Can you work these out from the model? Positions are in its coordinate system, mm. Face numbers are marked on the shaded views. A direction names the side the tool comes from. Give positions to 0.01 mm unless a question says otherwise; leave off trailing zeros. Write each loop counter-clockwise with the first axis right and the second up, starting at its lowest first coordinate (ties: lowest second). Pieces come first, ordered by that corner, then holes.
1. If I drill on probe 1 along X at (y, z) = (0, 0) (3 decimals); probe 2 along X at (y, z) = (-6, 1.75); probe 3 along Z at (x, y) = (-25.4, -0.5) (3 decimals), over which ranges is the centre line in solid material (lowest first)?
2. Suppose I cut it at C-C (x = 1.5). Please give me the cut outline in (y, z) (3 decimals), and give its area (3 significant figures).
3. Suppose I cut it at A-A (y = -7). Please give me the cut outline in (x, z), and give its area (3 significant figures).
4. Suppose I cut it at D-D (y = 0). Give the number of separate pieces and of enclosed holes in the cut face, and give its area (3 significant figures).
5. On a 3-axis mill with a long thin cutter (end or side, diameter ignored), from which of +Z, -Z, +X, -X, +Y, -Y can I reach the whole of each face in a straight line? I mean the marked faces 1, 2 and 3. Say none if no direction works.
6. Thinking about a two-plate mould opening in Z: for the marked faces 4 and 5, which applies, pulls with the +Z half, pulls with the -Z half, needs draft (parallel to the pull), parting line crosses it, or undercut?
7. I'm going to push flat-ended pins straight in: pin 1 (5.5 mm diameter, centred on x = -25.4, z = 0, fed in from +Y); pin 2 (5 mm diameter, centred on x = -26.5, z = -1, fed in from +Y); pin 3 (11.5 mm diameter, centred on x = 0, z = 0, fed in from +Y); pin 4 (4 mm diameter, centred on x = 2.5, y = 6.5, fed in from +Z). Where does each tip first touch, or does it pass through?
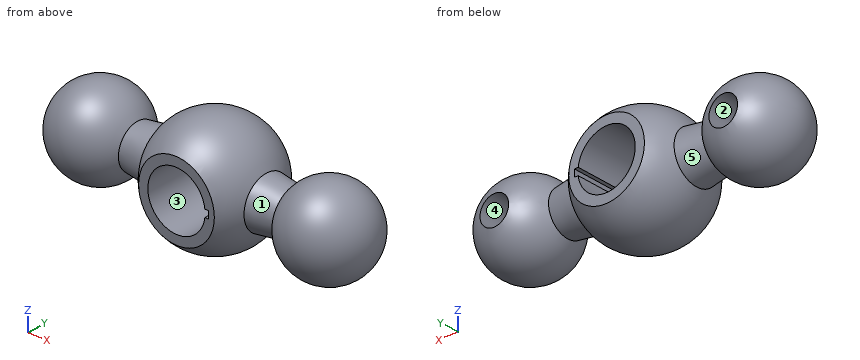
```python
from build123d import *
from build123d import SkipClean  # not in build123d's __all__

# Parameters (mm, degrees)
F8_W          = 16.8005208253
F8_H          = 3.175
F1_DEPTH      = 12.701
F1_DEPTH_BACK = 12.701
F3_DEPTH      = 19.05
F5_R          = 3.175
F6_DEPTH      = 13.255625


with BuildPart() as f7:
    # F0 (on Top) → F7 (revolve)
    with BuildSketch(Plane.XY):
        with BuildLine():
            Line((17.151108029, 4.7625), (11.4200738149, 5.55625))
            ThreePointArc((11.4200738149, 5.55625), (0, 12.7), (-11.4200738149, 5.55625))
            Line((-11.4200738149, 5.55625), (-17.151108029, 4.7625))
            ThreePointArc((-17.151108029, 4.7625), (-27.8652514046, 9.2004434954), (-34.925, 0))
            Line((-34.925, 0), (34.925, 0))
            ThreePointArc((34.925, 0), (27.8652514046, 9.2004434954), (17.151108029, 4.7625))
        make_face()
    revolve(axis=Axis((0, 0, 0), (1, 0, 0)))

    # F8 (on Top) → F1 (cut, two sides)
    with BuildSketch(Plane.XY) as f1_sk:
        with Locations((0, 11.1125)):
            Rectangle(F8_W, F8_H)
        with Locations((0, -11.1125)):
            Rectangle(F8_W, F8_H)
    with SkipClean():  # cleaning this boolean's faces spoils the solid; the shape is the same uncleaned
        extrude(amount=F1_DEPTH, mode=Mode.SUBTRACT)
        extrude(f1_sk.sketch, amount=-F1_DEPTH_BACK, mode=Mode.SUBTRACT)

    # F2 (on face) → F3 (cut, through all)
    with BuildSketch(Plane.XZ.offset(9.525)):
        with BuildLine():
            ThreePointArc((6.3001953095, -0.79375), (6.3375365962, -0.3976554946), (6.35, 0))
            ThreePointArc((6.35, 0), (6.3375365962, 0.3976554946), (6.3001953095, 0.79375))
            ThreePointArc((6.3001953095, 0.79375), (-6.35, 0), (6.3001953095, -0.79375))
        make_face()
        with BuildLine():
            ThreePointArc((6.3001953095, 0.79375), (6.3375365962, 0.3976554946), (6.35, 0))
            ThreePointArc((6.35, 0), (6.3375365962, -0.3976554946), (6.3001953095, -0.79375))
            Line((6.3001953095, -0.79375), (7.14375, -0.79375))
            Line((7.14375, -0.79375), (7.14375, 0.79375))
            Line((7.14375, 0.79375), (6.3001953095, 0.79375))
        make_face()
    with SkipClean():  # cleaning this boolean's faces spoils the solid; the shape is the same uncleaned
        extrude(amount=-F3_DEPTH, mode=Mode.SUBTRACT)

    # F5 (on plane+point) → F6 (cut)
    with BuildSketch(Plane.XZ.offset(-9.525)):
        with Locations((25.4, 0)):
            Circle(F5_R)
        with Locations((-25.4, 0)):
            Circle(F5_R)
    extrude(amount=F6_DEPTH, mode=Mode.SUBTRACT)


solid = f7.part
```
Checks:
1. probe 1: x = -34.925 to -28.575, -22.225 to -6.35, 7.144 to 22.225, 28.575 to 34.925
1. probe 2: x = -32.59 to -18.21, -11.06 to -6.1, 6.1 to 11.06, 18.21 to 32.59
1. probe 3: z = -9.512 to -3.175, 3.175 to 9.512
2. outline: (-9.525, -8.265) arc R12.611 ccw to (9.525, -8.265) - (9.525, -6.17) - (-9.525, -6.17) - close; (-9.525, 6.17) - (9.525, 6.17) - (9.525, 8.265) arc R12.611 ccw to (-9.525, 8.265) - close
2. area: 195 mm2
3. outline: circle Ø12.92 at (-25.4, 0); circle Ø21.19 at (0, 0); circle Ø12.92 at (25.4, 0); hole (6.3, -0.79) - (7.14, -0.79) - (7.14, 0.79) - (6.3, 0.79) arc R6.35 ccw (long way) to start
3. area: 487 mm2
4. separate pieces: 1
4. enclosed holes: 3
4. area: 968 mm2
5. face 1: none
5. face 2: +Y
5. face 3: +Y, -Y
6. face 4: undercut
6. face 5: parting line crosses it
7. pin 1: stops at y = -3.73
7. pin 2: stops at y = 8.98
7. pin 3: passes through
7. pin 4: stops at z = 11.69
